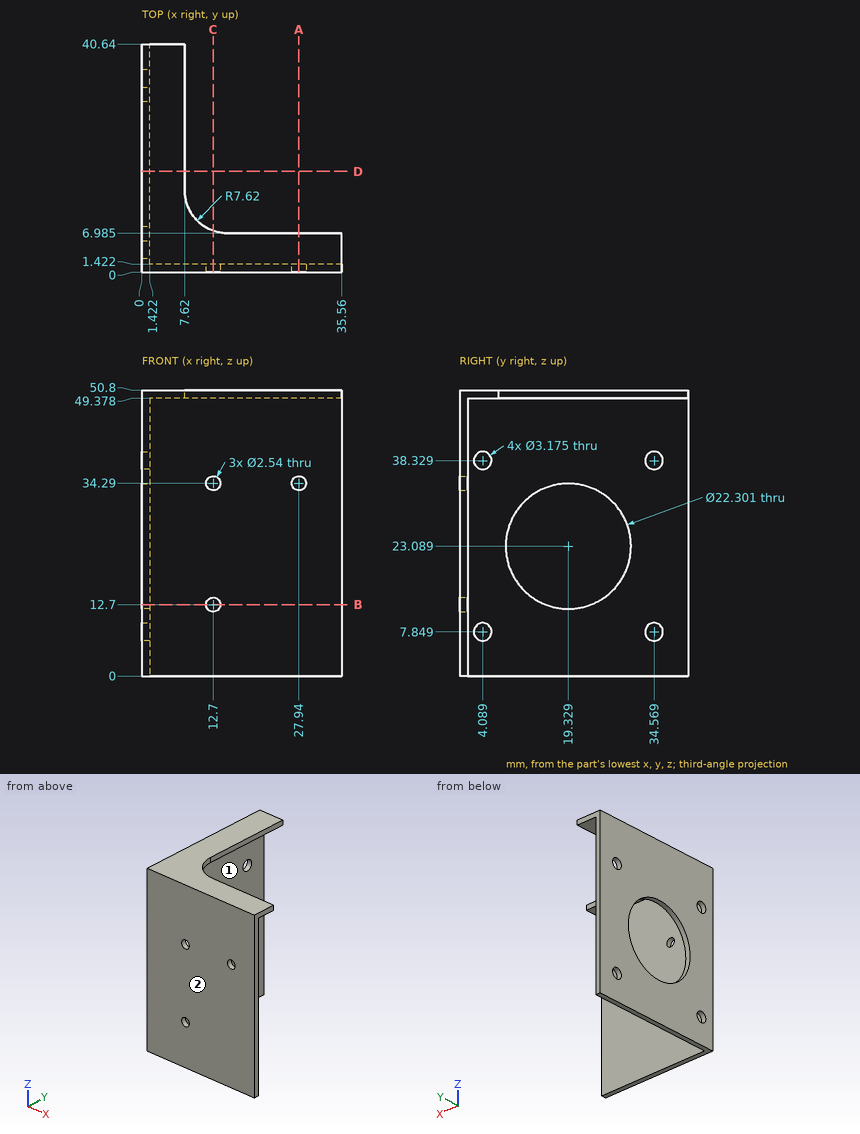
The drawing under review shows one solid part. Ordinate dimensions are in mm from its lowest x, y, z. A direction names the side the tool comes from. Round coordinates to 2 decimals unless told otherwise and drop trailing zeros. Write each loop counter-clockwise with the first axis right and the second up, starting at its lowest first coordinate (ties: lowest second). Pieces come first, ordered by that corner, then holes. Notation, with made-up numbers: (88, 68) -> (104, 68) arc R18 ccw to (104, 85) -> close; hole circle Ø9 at (57, 13.5). An arc over 180 degrees is marked (long way). One line per question, with ' | ' between items.
(1) Wall thickness on line 1 (Z direction, x = 12, y = 1); line 2 (Y direction, x = 20, z = 38.5): over which ranges is each line inside the solid? List them lowest first. Write a range as [from, to].
Result sheet:
line 1: [0, 11.64], [13.76, 33.23], [35.35, 50.8] | line 2: [0, 1.42]
(2) Take a section at D-D, the plane y = 18. State the section outline as (x, z) points.
Result sheet:
outline: (0, 0) -> (1.42, 0) -> (1.42, 12.02) -> (0, 12.02) -> close; (0, 34.16) -> (1.42, 34.16) -> (1.42, 49.38) -> (7.62, 49.38) -> (7.62, 50.8) -> (0, 50.8) -> close
(3) Insertion check: P1, Ø5, axis at x = 29.5, z = 42, coming from the +Y side; P2, Ø3, axis at y = 24.5, z = 12, coming from the +X side; P3, Ø2, axis at x = 27.94, z = 34.29, coming from the -Y side; P4, Ø10, axis at x = 12.5, y = 14.5, coming from the -Z side. Each pin has a flat end and moves straight along its axis. Give the tip position at first contact, or say it passes through.
Result sheet:
P1: y = 1.42 | P2: x = 1.42 | P3: through | P4: z = 49.38
(4) Machinability: for the marked faces 1 and 2, which of the approach directions +Z, -Z, +X, -X, +Y, -Y give a long, thin tool a straight path to every point of the face, cutting with its end or side? Answer none if there is none.
Result sheet:
face 1: -Z, +X, +Y | face 2: +Z, -Z, +X, -X, -Y
(5) Take a section at A-A, the plane x = 27.94. State the section outline as (y, z) points (1 decimal).
Result sheet:
outline: (0, 0) -> (1.4, 0) -> (1.4, 33) -> (0, 33) -> close; (0, 35.6) -> (1.4, 35.6) -> (1.4, 49.4) -> (7, 49.4) -> (7, 50.8) -> (0, 50.8) -> close
(6) Take a section at B-B, the plane z = 12.7. State the section outline as (x, y) points.
Result sheet:
outline: (0, 0) -> (11.43, 0) -> (11.43, 1.42) -> (1.42, 1.42) -> (1.42, 15.28) -> (0, 15.28) -> close; (0, 23.38) -> (1.42, 23.38) -> (1.42, 40.64) -> (0, 40.64) -> close; (13.97, 0) -> (35.56, 0) -> (35.56, 1.42) -> (13.97, 1.42) -> close
(7) Take a section at C-C, the plane x = 12.7. State the section outline as (y, z) points.
Result sheet:
outline: (0, 0) -> (1.42, 0) -> (1.42, 11.43) -> (0, 11.43) -> close; (0, 13.97) -> (1.42, 13.97) -> (1.42, 33.02) -> (0, 33.02) -> close; (0, 35.56) -> (1.42, 35.56) -> (1.42, 49.38) -> (7.42, 49.38) -> (7.42, 50.8) -> (0, 50.8) -> close
